For this review, take the finished solid that the model builds, in its own axes (mm). A direction names the side the tool comes from. Coordinates: 2 decimals unless noted, no trailing zeros. Write each loop counter-clockwise with the first axis right and the second up, starting at its lowest first coordinate (ties: lowest second). Pieces come first, ordered by that corner, then holes.
1) We need section D-D on y = 6.25. Write out the cut boundary in (x, z) (1 decimal).
2) We need section B-B on z = 11.43. Write out the cut boundary in (x, y) (3 decimals).
3) For faces 4 (the face through (19.443, 2, 11)), 5 (the face through (-3.6, 6.4, 19.8)), list the 3-axis set-ups (+Z, -Z, +X, -X, +Y, -Y) from which the entire face can be reached by the end or side of a thin tool; tool diameter is ignored.
4) We need section C-C on x = 3.5. Write out the cut boundary in (y, z) (3 decimals), then the cut area to 3 significant figures.
5) To check wall thickness, follow line 1 along X through (y, z) = (0.85, 11.43); line 2 along X through (y, z) = (3.75, 17.25); line 3 along Y through (x, z) = (8.5, 13.25). State the ranges of each line that lie inside material, in increasing order.
6) Insertion check: P1, Ø4, axis at x = 4.84, z = 11.43, coming from the -Y side; P2, Ø1.5, axis at y = 5, z = 19.5, coming from the -X side; P3, Ø6, axis at x = 6.5, z = 13.5, coming from the +Y side. Each pin has a flat end and moves straight along its axis. Give the tip position at first contact, or say it passes through.
7) Mouldability with a two-part tool opening along X and no side actions: class faces 1 (the face through (-6.592, 3, 11)), 2 (the face through (2, 3.81, 12)), 3 (the face through (9.042, 6.341, 0.626)) as pulls with the +X half, pulls with the -X half, needs draft (parallel to the pull), parting line crosses it, or undercut.
8) We need section A-A on y = 2.25. Write out the cut boundary in (x, z), then the cut area to 3 significant figures.
from build123d import *

# Parameters (mm, degrees)
F1_DEPTH  = 22.86
F2_SIZE2  = 31.75
F2_SIZE   = 5.08
F3_SIZE   = 5.08
F5_DEPTH  = 3.81
F6_SIZE   = 1.27
F7_R      = 2.38125
F8_DEPTH  = 25.4
F9_R      = 6.0325
F9_R_2    = 2.38125
F10_DEPTH = 3.175


with BuildPart() as f1:
    # F0 (on Top) → F1 (new body)
    with BuildSketch(Plane.XY):
        Polygon((-6.5924515948, 3.175), (-6.5924515948, 0), (19.4425484052, 0), (19.4425484052, 3.81), (48.4711198338, 3.81), (48.4711198338, 0), (51.6461198338, 0), (51.6461198338, 6.985), (16.2675484052, 6.985), (16.2675484052, 3.175), align=None)
    extrude(amount=F1_DEPTH)

    # F2
    f2_edges = [f1.edges().sort_by_distance(p)[0] for p in [
        (51.64612, 3.4925, 22.86),
        (51.64612, 3.4925, 0),
    ]]
    f2_side = f1.faces().sort_by_distance((51.64612, 3.4925, 11.43))[0]
    chamfer(f2_edges, length=F2_SIZE, length2=F2_SIZE2, reference=f2_side)

    # F3
    f3_edges = [f1.edges().sort_by_distance(p)[0] for p in [
        (-6.592452, 1.5875, 0),
        (-6.592452, 1.5875, 22.86),
    ]]
    chamfer(f3_edges, length=F3_SIZE)

    # F4 (on face) → F5 (join, through all)
    with BuildSketch(Plane(origin=(0, 3.175, 0), x_dir=(-1, 0, 0), z_dir=(0, 1, 0))):
        Polygon((1.5124515948, 0), (6.5924515948, 5.08), (6.5924515948, 17.78), (1.5124515948, 22.86), (-16.2675484052, 22.86), (-16.2675484052, 0), align=None)
    extrude(amount=F5_DEPTH)

    # F6
    f6_edges = [f1.edges().sort_by_distance(p)[0] for p in [
        (51.64612, 6.985, 11.43),
        (35.77112, 6.985, 20.32),
        (9.191834, 6.985, 22.86),
        (-4.052452, 6.985, 20.32),
        (-6.592452, 6.985, 11.43),
        (-4.052452, 6.985, 2.54),
        (9.191834, 6.985, 0),
        (35.77112, 6.985, 2.54),
    ]]
    chamfer(f6_edges, length=F6_SIZE)

    # F7 (on face) → F8 (cut)
    with BuildSketch(Plane.XZ):
        with Locations((4.8375484052, 11.43)):
            Circle(F7_R)
    extrude(amount=-F8_DEPTH, mode=Mode.SUBTRACT)

    # F9 (on face) → F10 (cut)
    with BuildSketch(Plane(origin=(0, 6.985, 0), x_dir=(-1, 0, 0), z_dir=(0, 1, 0))):
        with Locations((-4.8375484052, 11.43)):
            Circle(F9_R)
        with Locations((-4.8375484052, 11.43)):
            Circle(F9_R_2, mode=Mode.SUBTRACT)
    extrude(amount=-F10_DEPTH, mode=Mode.SUBTRACT)


solid = f1.part
Result:
1. outline: (-6.1, 5.3) - (-1.3, 0.5) - (19.9, 0.5) - (51.1, 5.5) - (51.1, 17.3) - (19.9, 22.3) - (-1.3, 22.3) - (-6.1, 17.6) - close; hole circle Ø12.1 at (4.8, 11.4)
2. outline: (-6.592, 0) - (2.456, 0) - (2.456, 3.81) - (-1.195, 3.81) - (-1.195, 6.985) - (-5.322, 6.985) - (-6.592, 5.715) - close; (7.219, 0) - (19.443, 0) - (19.443, 3.81) - (48.471, 3.81) - (48.471, 0) - (51.646, 0) - (51.646, 5.715) - (50.376, 6.985) - (10.87, 6.985) - (10.87, 3.81) - (7.219, 3.81) - close
3. face 4: +Z, -Z, -Y
3. face 5: +Z, -X, +Y
4. outline: (0, 0) - (5.715, 0) - (6.985, 1.27) - (6.985, 5.548) - (3.81, 5.548) - (3.81, 9.46) - (0, 9.46) - close; (0, 13.4) - (3.81, 13.4) - (3.81, 17.312) - (6.985, 17.312) - (6.985, 21.59) - (5.715, 22.86) - (0, 22.86) - close
4. area: 106 mm2
5. line 1: x = -6.59 to 2.46, 7.22 to 19.44, 48.47 to 51.65
5. line 2: x = -6.59 to 19.44, 48.47 to 51.65
5. line 3: y = 0 to 3.81
6. P1: passes through
6. P2: stops at x = -5.62
6. P3: stops at y = 3.81
7. face 1: pulls with the -X half
7. face 2: undercut
7. face 3: needs draft
8. outline: (-6.59, 5.08) - (-1.51, 0) - (19.44, 0) - (19.44, 22.86) - (-1.51, 22.86) - (-6.59, 17.78) - close; (48.47, 4.57) - (51.65, 5.08) - (51.65, 17.78) - (48.47, 18.29) - close; hole circle Ø4.76 at (4.84, 11.43)
8. area: 593 mm2
